Autodesk Inventor part; units mm, degrees
sketch "Sketch5" plane through (0, 0, 0) normal (0, 0, 1) x (1, 0, 0)
  line L0 (-500, -250) -> (500, -250)
  line L1 (500, -250) -> (500, 250)
  line L2 (500, 250) -> (-500, 250)
  line L3 (-500, 250) -> (-500, -250)
  line L4 (-500, -250) -> (500, 250) construction
  line L5 (500, -250) -> (-500, 250) construction
  point P0 (0, 0)
  dimension "d11" = 1000
  dimension "d12" = 500
extrude "Extrusion3" add sketch "Sketch5" along normal mid plane 500
sketch "Sketch6" plane through (500, -250, 250) normal (1, 0, 0) x (0, 0, -1)
  line L0 (0, 0) -> (0, 500) construction
  line L1 (500, 0) -> (500, 500) construction
  line L2 (0, 52.5521) -> (500, 0)
  line L3 (500, 0) -> (0, 0)
  line L4 (0, 0) -> (0, 52.5521)
  point P0 (250, 250)
  dimension "d15" = 6
extrude "Extrusion4" cut sketch "Sketch6" against normal up to next
mirror "Mirror2" about plane through (0, 0, 0) normal (0, 1, 0) of "Extrusion4"
sketch "Sketch7" plane through (-500, -250, -250) normal (0, -0.9945, 0.1045) x (1, 0, 0)
  line L0 (0, 402.7541) -> (1000, 315.2655)
  line L1 (1000, 502.7541) -> (1000, 0) construction
  line L2 (0, 502.7541) -> (1000, 502.7541) construction
  line L3 (0, 0) -> (0, 502.7541) construction
  point P0 (500, 274.7626)
  dimension "d18" = 5
  dimension "d19" = 100
sketch "Sketch8" plane through (-500, -250, -250) normal (0, -0.9945, 0.1045) x (1, 0, 0)
  line L0 (0, 0) -> (0, 502.7541) construction
  line L1 (0, 90) -> (1000, 212.7846)
  line L2 (1000, 502.7541) -> (1000, 0) construction
  line L3 (1000, 0) -> (0, 0) construction
  point P0 (500, 274.7626)
  dimension "d20" = 7
  dimension "d21" = 90
properties part number "Telaio"
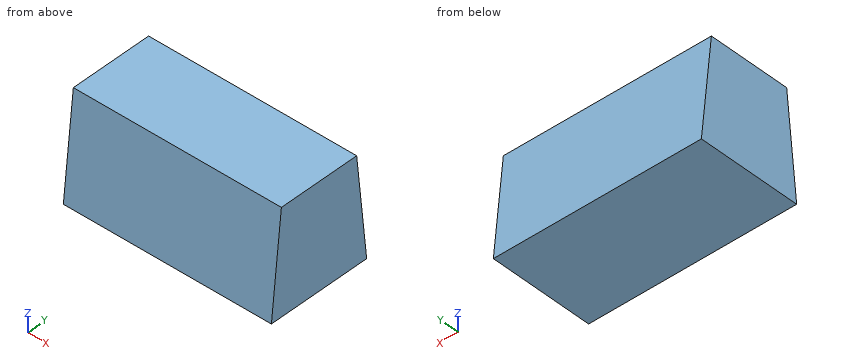
The model under review builds one solid part; all positions refer to its coordinate system, in mm. Round coordinates to 2 decimals unless told otherwise and drop trailing zeros. Order: outer loops, then holes, each group sorted by start corner. A loop starts at its lowest first (then second) coordinate and runs counter-clockwise, first axis right, second up. Notation, with made-up numbers: (-20.5, 58) -> (32.5, 58) arc R28 ccw to (32.5, 86) -> close; hole circle Ø9 at (35.5, 50). An arc over 180 degrees is marked (long way). Use CSV: the item, a comma, the result in double quotes. Start each with the question number.
(1) Insertion check: pin 1 (8 mm diameter, centred on x = 148, z = 75, fed in from +Y); pin 2 (3 mm diameter, centred on x = -370, z = -99.5, fed in from +Y); pin 3 (4 mm diameter, centred on x = -100.5, z = -34.5, fed in from +Y). Each pin has a flat end and moves straight along its axis. Give the tip position at first contact, or say it passes through.
(2) Consider section B-B on z = 75. Write out the cut boundary in (x, y).
(3) Wall thickness on probe 1 along Y at (x, z) = (321, -27.5); probe 2 along Y at (x, z) = (164, -205): over which ranges is each line inside the solid? List them lowest first. Write a range as from..to.
(4) Consider section A-A on x = -124. Write out the cut boundary in (y, z), and give its area (3 significant figures).
Responses:
1,pin 1,"y = 216.26"
1,pin 2,"y = 234.34"
1,pin 3,"y = 227.56"
2,outline,"(-500, -215.84) -> (500, -215.84) -> (500, 215.84) -> (-500, 215.84) -> close"
3,probe 1,"-226.61..226.61"
3,probe 2,"-245.27..245.27"
4,outline,"(-250, -250) -> (250, -250) -> (197.45, 250) -> (-197.45, 250) -> close"
4,area,"224,000 mm²"
